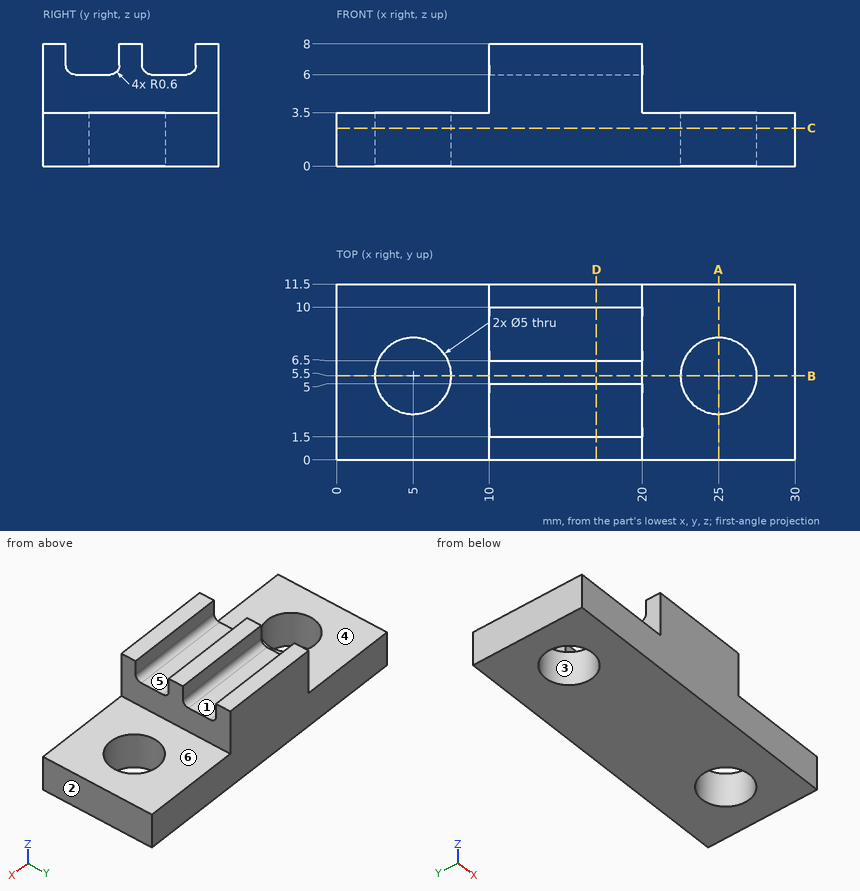
Source: three-view drawing plus pictorial views. Frame: mm from the lowest corner of the part. A direction names the side the tool comes from. Give positions to 0.01 mm unless a question says otherwise; leave off trailing zeros. Loops run counter-clockwise (first coordinate to the right, second up) from the corner with the lowest first, then second, coordinate; pieces in that order, holes last. Notation, with made-up numbers: M -8,6 L 34,6 A25 ccw 34,27 Z; hole C 60,19.25 d6. An arc over 180 degrees is marked long. Put each result on its own line as item: value.
Q1. Section D-D (x = 17). Return the cut outline in (y, z), and give its area (3 significant figures).
Response values:
outline: M 0,0 L 11.5,0 L 11.5,8 L 10,8 L 10,6.6 A0.6 cw 9.4,6 L 7.1,6 A0.6 cw 6.5,6.6 L 6.5,8 L 5,8 L 5,6.6 A0.6 cw 4.4,6 L 2.1,6 A0.6 cw 1.5,6.6 L 1.5,8 L 0,8 Z
area: 78.3 mm²
Q2. Section C-C (z = 2.5). Return the cut outline in (x, y).
Response values:
outline: M 0,0 L 30,0 L 30,11.5 L 0,11.5 Z; hole C 5,5.5 d5; hole C 25,5.5 d5
Q3. Line query: probe 1 along Y at (x, z) = (25, 0.9); probe 2 along X at (y, z) = (9.25, 4.75); probe 3 along Z at (x, y) = (18, 2.75). Output: solid intervals per line, ascending. Write a range as [from, to].
Response values:
probe 1: y = [0, 3], [8, 11.5]
probe 2: x = [10, 20]
probe 3: z = [0, 6]
Q4. Mould query, pull axis X, two halves, no side actions, for the marked faces 1, 2 and 3. Classes: released by +X, released by -X, zero draft, split by the parting line, or undercut.
Response values:
face 1: zero draft
face 2: released by +X
face 3: undercut
Q5. Section A-A (x = 25). Return the cut outline in (y, z), and give its area (4 significant figures).
Response values:
outline: M 0,0 L 3,0 L 3,3.5 L 0,3.5 Z; M 8,0 L 11.5,0 L 11.5,3.5 L 8,3.5 Z
area: 22.75 mm²
Q6. Section B-B (y = 5.5). Return the cut outline in (x, z).
Response values:
outline: M 0,0 L 2.5,0 L 2.5,3.5 L 0,3.5 Z; M 7.5,0 L 22.5,0 L 22.5,3.5 L 20,3.5 L 20,8 L 10,8 L 10,3.5 L 7.5,3.5 Z; M 27.5,0 L 30,0 L 30,3.5 L 27.5,3.5 Z
Q7. Pin query (flat end, axial travel): P1, Ø0.7, axis at x = 14, y = 3, coming from the +Z side; P2, Ø2.5, axis at x = 16, y = 8, coming from the +Z side; P3, Ø2, axis at y = 5, z = 6.5, coming from the -X side. Return the tip coordinate at first contact, or that it passes through.
Response values:
P1: stops at z = 6
P2: stops at z = 6.11
P3: stops at x = 10
Q8. Reachability of the marked faces 4, 5 and 6 from +Z, -Z, +X, -X, +Y, -Y: full face, straight path, thin tool, end or side. Return the list, or none.
Response values:
face 4: +Z, -X, +Y, -Y
face 5: +Z, +X, -X
face 6: +Z, +X, +Y, -Y
